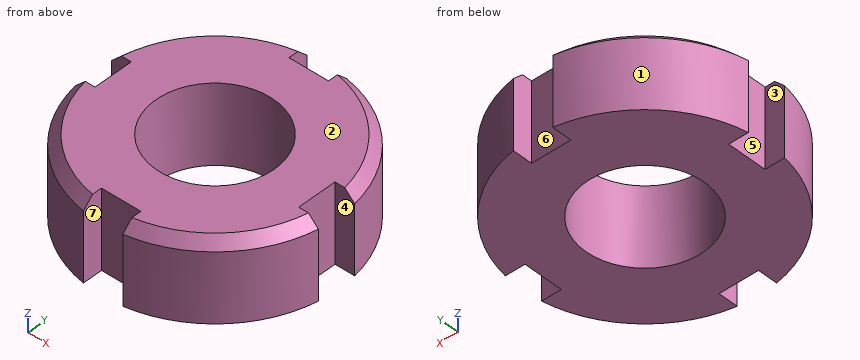
from build123d import *

# Parameters (mm, degrees)
SKETCH1_R           = 12.5
BOSS_EXTRUDE1_DEPTH = 8
CUT_EXTRUDE1_DEPTH  = 20.403607912
SKETCH3_R           = 6
CUT_EXTRUDE2_DEPTH  = 20.19635382
CHAMFER1_SIZE       = 1


with BuildPart() as part:
    # Sketch1 → Boss-Extrude1 (new body)
    with BuildSketch(Plane.XY):
        Circle(SKETCH1_R)
    extrude(amount=BOSS_EXTRUDE1_DEPTH)

    # Sketch2 → Cut-Extrude1 (cut, through all)
    with BuildSketch(Plane.XY.offset(8)):
        with BuildLine():
            Line((-2, 12.338962679), (-2, 10.338962679))
            Line((-2, 10.338962679), (2, 10.338962679))
            Line((2, 10.338962679), (2, 12.338962679))
            ThreePointArc((2, 12.338962679), (0, 12.5), (-2, 12.338962679))
        make_face()
        with BuildLine():
            Line((12.338962679, 2), (10.338962679, 2))
            Line((10.338962679, 2), (10.338962679, -2))
            Line((10.338962679, -2), (12.338962679, -2))
            ThreePointArc((12.338962679, -2), (12.5, 0), (12.338962679, 2))
        make_face()
        with BuildLine():
            Line((2, -12.338962679), (2, -10.338962679))
            Line((2, -10.338962679), (-2, -10.338962679))
            Line((-2, -10.338962679), (-2, -12.338962679))
            ThreePointArc((-2, -12.338962679), (0, -12.5), (2, -12.338962679))
        make_face()
        with BuildLine():
            Line((-12.338962679, -2), (-10.338962679, -2))
            Line((-10.338962679, -2), (-10.338962679, 2))
            Line((-10.338962679, 2), (-12.338962679, 2))
            ThreePointArc((-12.338962679, 2), (-12.5, 0), (-12.338962679, -2))
        make_face()
    extrude(amount=-CUT_EXTRUDE1_DEPTH, mode=Mode.SUBTRACT)

    # Sketch3 → Cut-Extrude2 (cut, through all)
    with BuildSketch(Plane.XY.offset(8)):
        Circle(SKETCH3_R)
    extrude(amount=-CUT_EXTRUDE2_DEPTH, mode=Mode.SUBTRACT)

    # Chamfer1
    chamfer1_edges = [part.edges().sort_by_distance(p)[0] for p in [
        (-8.838834765, 8.838834765, 8),
        (-8.838834765, -8.838834765, 8),
        (8.838834765, -8.838834765, 8),
        (8.838834765, 8.838834765, 8),
    ]]
    chamfer(chamfer1_edges, length=CHAMFER1_SIZE)


solid = part.part
Could you check a few things on this model? Use its own coordinates, in mm. Face numbers are marked on the shaded views. A direction names the side the tool comes from. Give positions to 0.01 mm unless a question says otherwise; leave off trailing zeros. Write each loop counter-clockwise with the first axis right and the second up, starting at its lowest first coordinate (ties: lowest second). Pieces come first, ordered by that corner, then holes. Notation, with made-up numbers: (32.5, 44.25) -> (37.5, 44.25) arc R5 ccw to (37.5, 49.25) -> close; hole circle Ø5 at (43, 72). An arc over 180 degrees is marked (long way). Write each question's results on one line, items separated by ' | '. Start each with the question number.
Q1. Which directions (+Z, -Z, +X, -X, +Y, -Y) give clear straight access to the entire face, cutting with the end or side of a thin tool? Please do the marked faces 5, 6 and 7.
Q2. I need wall thicknesses on probe 1 along Y at (x, z) = (0, 2); probe 2 along Y at (x, z) = (-3.5, 3.75); probe 3 along X at (y, z) = (10.75, 6.25). Which ranges of each line are inside material? Lowest first, please.
Q3. I'm going to push flat-ended pins straight in: pin 1 Ø1 at (x, z) = (-11, 3.5) entering from -Y; pin 2 Ø1 at (x, z) = (-11, 2) entering from +Y; pin 3 Ø3 at (x, z) = (-1, 3) entering from +Y; pin 4 Ø4.5 at (y, z) = (0, 2) entering from -X. Where does each tip first touch, or does it pass through?
Q4. Suppose I cut it at D-D, the plane z = 7.5. List the corners of the cut face in (x, y) for me, and give its area (3 significant figures).
Q5. Suppose I cut it at A-A, the plane y = 0. List the corners of the cut face in (x, z) for me, and give its area (3 significant figures).
Q6. Suppose I cut it at C-C, the plane z = 1.5. List the corners of the cut face in (x, y) for me.
Q7. We'd pull the mould along Y, two halves only. Please class the marked faces 1, 2, 3 and 4: +Y half, -Y half, draft (parallel to the pull), parting line (faces both ways), or undercut.
Outcome:
1) face 5: +Z, -Z, -X | face 6: +Z, -Z, +Y | face 7: +Z, -Z, -Y
2) probe 1: -10.34 to -6, 6 to 10.34 | probe 2: -12 to -4.87, 4.87 to 12 | probe 3: -6.38 to -2, 2 to 6.38
3) pin 1: y = -6.78 | pin 2: y = 6.78 | pin 3: y = 12.34 | pin 4: x = -12.34
4) outline: (-11.83, -2) arc R12 ccw to (-2, -11.83) -> (-2, -10.34) -> (2, -10.34) -> (2, -11.83) arc R12 ccw to (11.83, -2) -> (10.34, -2) -> (10.34, 2) -> (11.83, 2) arc R12 ccw to (2, 11.83) -> (2, 10.34) -> (-2, 10.34) -> (-2, 11.83) arc R12 ccw to (-11.83, 2) -> (-10.34, 2) -> (-10.34, -2) -> close; hole circle Ø12 at (0, 0) | area: 314 mm2
5) outline: (-10.34, 0) -> (-6, 0) -> (-6, 8) -> (-10.34, 8) -> close; (6, 0) -> (10.34, 0) -> (10.34, 8) -> (6, 8) -> close | area: 69.4 mm2
6) outline: (-12.34, -2) arc R12.5 ccw to (-2, -12.34) -> (-2, -10.34) -> (2, -10.34) -> (2, -12.34) arc R12.5 ccw to (12.34, -2) -> (10.34, -2) -> (10.34, 2) -> (12.34, 2) arc R12.5 ccw to (2, 12.34) -> (2, 10.34) -> (-2, 10.34) -> (-2, 12.34) arc R12.5 ccw to (-12.34, 2) -> (-10.34, 2) -> (-10.34, -2) -> close; hole circle Ø12 at (0, 0)
7) face 1: +Y half | face 2: draft | face 3: undercut | face 4: undercut
